The listing builds one solid part. Answer for the finished solid, in the listing's coordinates (mm). Face numbers are marked on the shaded views. A direction names the side the tool comes from. Give positions to 0.01 mm unless a question says otherwise; leave off trailing zeros. Loops run counter-clockwise (first coordinate to the right, second up) from the corner with the lowest first, then second, coordinate; pieces in that order, holes last. Notation, with made-up numbers: M 13,17.5 L 66,17.5 A28 ccw 66,42.5 Z; hole C 11.5,82 d5. An arc over 180 degrees is marked long. Use one line per item in the form item = value. Start each with the question number.
1. The part is cut by section C-C (z = 13.5). Write down the section's boundary in (x, y), and give its area (3 significant figures).
2. For the marked faces 1, 2, 3, 4 and 5, determine the directions among +Z, -Z, +X, -X, +Y, -Y from which every point of the face is accessible in a straight line to the end or side of a thin tool.
3. Each of these flat-tipped pins is pushed along its axis until it touches: pin 1 Ø25 at (y, z) = (31, 1.5) entering from +X; pin 2 Ø8 at (x, z) = (87.5, 20) entering from -Y; pin 3 Ø20 at (x, y) = (27, 39) entering from -Z. Where does it stop, or does it pass through?
4. The part is cut by section A-A (y = 64). Write down the section's boundary in (x, z), and give its area (3 significant figures).
5. The part is cut by section B-B (x = 26). Write down the section's boundary in (y, z), and give its area (3 significant figures).
6. Straight lines are drawn through the part: line 1 (Z direction, x = 56.5, y = 76.5); line 2 (X direction, y = 16, z = 25.5); line 3 (X direction, y = 39.5, z = 17). For each, find the intervals that lie inside material, in ascending order. Write a range as from..to.
7. The mould has two halves that part along Z. Classify the marked faces 6, 7 and 8: released by +Z, released by -Z, zero draft, split by the parting line, or undercut.
8. The part is cut by section D-D (x = 12). Write down the section's boundary in (y, z), and give its area (3 significant figures).
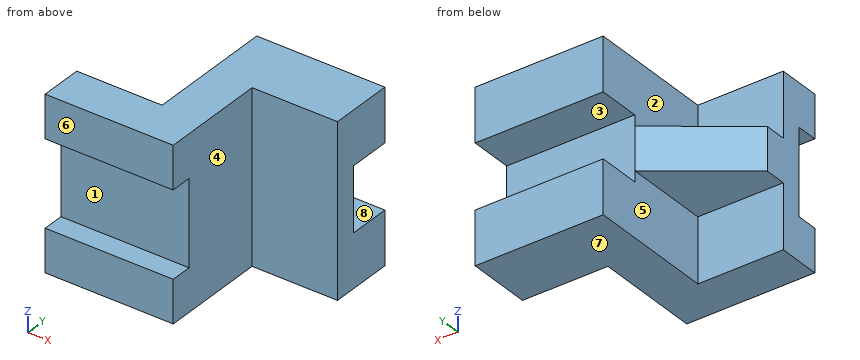
from build123d import *

# Parameters (mm, degrees)
BOSS_EXTRUDE1_DEPTH = 40
BOSS_EXTRUDE2_DEPTH = 10
SKETCH2_W           = 40
SKETCH2_H           = 10
SKETCH2_W_2         = 30
SKETCH2_H_2         = 20
CUT_EXTRUDE1_DEPTH  = 135.16407865


with BuildPart() as part:
    # Sketch1 → Boss-Extrude1 (new, symmetric)
    with BuildSketch(Plane.XY):
        Polygon((40, 20), (0, 20), (0, 0), (60, 0), (60, 50), (100, 50), (100, 80), (40, 80), align=None)
    extrude(amount=BOSS_EXTRUDE1_DEPTH, both=True)

    # Sketch1_3 → Boss-Extrude2 (add, symmetric)
    with BuildSketch(Plane.XY):
        Polygon((0, 30), (0, 20), (40, 20), (40, 60), align=None)
    extrude(amount=BOSS_EXTRUDE2_DEPTH, both=True)

    # Sketch2 → Cut-Extrude1 (cut, through all)
    with BuildSketch(Plane(origin=(0, 0, 0), x_dir=(0, 0, -1), z_dir=(1, 0, 0))):
        with Locations((0, 5)):
            Rectangle(SKETCH2_W, SKETCH2_H)
        with Locations((0, 70)):
            Rectangle(SKETCH2_W_2, SKETCH2_H_2)
    extrude(amount=CUT_EXTRUDE1_DEPTH, mode=Mode.SUBTRACT)


solid = part.part
Derived:
q1.outline = M 0,10 L 60,10 L 60,50 L 100,50 L 100,60 L 40,60 L 40,20 L 0,20 Z
q1.area = 1,800 mm2
q2.face_1 = +X, -X, -Y
q2.face_2 = +Z, -X, +Y
q2.face_3 = +X, -X, +Y
q2.face_4 = +Z, -Z, +X, -Y
q2.face_5 = -Z, -X, +Y
q3.pin_1 = 60
q3.pin_2 = 50
q3.pin_3 = -10
q4.outline = M 40,-40 L 100,-40 L 100,-15 L 40,-15 Z; M 40,15 L 100,15 L 100,40 L 40,40 Z
q4.area = 3,000 mm2
q5.outline = M 0,-40 L 20,-40 L 20,-10 L 49.5,-10 L 49.5,10 L 20,10 L 20,40 L 0,40 L 0,20 L 10,20 L 10,-20 L 0,-20 Z
q5.area = 1,790 mm2
q6.line_1 = -40..-15, 15..40
q6.line_2 = 0..60
q6.line_3 = 40..60
q7.face_6 = zero draft
q7.face_7 = released by -Z
q7.face_8 = undercut
q8.outline = M 0,-40 L 20,-40 L 20,-10 L 39,-10 L 39,10 L 20,10 L 20,40 L 0,40 L 0,20 L 10,20 L 10,-20 L 0,-20 Z
q8.area = 1,580 mm2
